Here's how the part is built. I have some questions about the finished solid (model axes, mm). A direction names the side the tool comes from. Round coordinates to 2 decimals unless told otherwise and drop trailing zeros. Loops run counter-clockwise (first coordinate to the right, second up) from the corner with the lowest first, then second, coordinate; pieces in that order, holes last. Notation, with made-up numbers: (42.5, -11.5) -> (90.5, -11.5) arc R15 cw to (90.5, 11.5) -> close; hole circle Ø8 at (13.25, -3.5). An arc over 180 degrees is marked (long way). One line per item, written item: value. Start each with the question number.
```python
from build123d import *

# Parameters (mm, degrees)
BOSS_EXTRUDE1_DEPTH = 8
SKETCH3_R           = 2.55
BOSS_EXTRUDE2_DEPTH = 1.5
CUT_EXTRUDE1_START  = -9.6
SKETCH3_3_R         = 2.55
CUT_EXTRUDE1_DEPTH  = 1.75


with BuildPart() as part:
    # Sketch1 → Boss-Extrude1 (new body)
    with BuildSketch(Plane(origin=(0, -47.198737708, 1.758e-06), x_dir=(1, 0, 0), z_dir=(1.517238059440084e-15, 0.9999999999999994, -3.725290356966477e-08))):
        with BuildLine():
            Line((7.999998093, 18.45445013), (7.999998093, 8.85445013))
            Line((7.999998093, 8.85445013), (14.894330873, 8.85445013))
            ThreePointArc((14.894330873, 8.85445013), (13.486635699, 16.156799215), (20.149998093, 12.85445013))
            ThreePointArc((20.149998093, 12.85445013), (19.302347178, 10.341087736), (17.105665312, 8.85445013))
            Line((17.105665312, 8.85445013), (23.999998093, 8.85445013))
            Line((23.999998093, 8.85445013), (23.999998093, 18.45445013))
            Line((23.999998093, 18.45445013), (7.999998093, 18.45445013))
        make_face()
    extrude(amount=BOSS_EXTRUDE1_DEPTH)

    # Sketch2 → Cut-Revolve1 (revolve, cut)
    with BuildSketch(Plane.ZY.offset(-15.999998093)):
        Polygon((-8.854448524, -44.263738058), (-8.619448462, -44.767697268), (-8.619448461, -44.798738029), (-8.854448524, -44.798738345), align=None)
    revolve(axis=Axis((15.999998093, -46.259040624, -12.929448669), (0, -1, 0)), mode=Mode.SUBTRACT)

    # Sketch3 → Boss-Extrude2 (add)
    with BuildSketch(Plane(origin=(0, -3.3e-07, -8.85445013), x_dir=(1, 0, 0), z_dir=(0, 3.725290356966478e-08, 0.9999999999999994))):
        with Locations(Location((11.999998093, -43.198737708, 0), (0, 0, 90))):
            Circle(SKETCH3_R)
        with Locations(Location((19.999998093, -43.198737708, 0), (0, 0, 90))):
            Circle(SKETCH3_R)
    extrude(amount=BOSS_EXTRUDE2_DEPTH)

    # Sketch3<3> → Cut-Extrude1 (cut)
    with BuildSketch(Plane(origin=(0, -3.3e-07, -8.85445013), x_dir=(1, 0, 0), z_dir=(0, 3.725290356966478e-08, 0.9999999999999994)).offset(CUT_EXTRUDE1_START)):
        with Locations(Location((11.999998093, -43.198737708, 0), (0, 0, 90))):
            Circle(SKETCH3_3_R)
        with Locations(Location((19.999998093, -43.198737708, 0), (0, 0, 90))):
            Circle(SKETCH3_3_R)
    extrude(amount=CUT_EXTRUDE1_DEPTH, mode=Mode.SUBTRACT)


solid = part.part
```
Q1. Will this pin go through, and if not, where does the flat tip stop? P1, Ø2.5, axis at x = 12, y = -43, coming from the -Z side.
Q2. Which directions (+Z, -Z, +X, -X, +Y, -Y) give clear straight access to the entire face, cutting with the end or side of a thin tool? Please do faces 1 (the flat face through (20, -43, -7.354)), 2 (the cylindrical face through (17.47, -43.53, -17.59)), 3 (the cylindrical face through (11.234, -40.766, -8.115)).
Q3. I want a section at D-D on x = 20.5. Please give me the cut outline in (y, z), plus the area to 3 significant figures.
Q4. If we mould it in two halves opening along Z, with no side actions, what happens to faces 4 (the flat face through (18, -47.199, -17)), 5 (the conical face through (15.83, -44.41, -17.07)), 6 (the flat face through (23, -43, -8.854))? For each: released by +Z, released by -Z, zero draft, split by the parting line, or undercut.
Q5. If I drill on line 1 along Z through (x, y) = (21.5, -42.75); line 2 along Z through (x, y) = (10.5, -40.25); line 3 along X through (y, z) = (-45.25, -11.25), over which ranges is the centre line in solid material (lowest first)?
Q6. I want a section at B-B on x = 9.75. Please give me the cut outline in (y, z).
Q7. I want a section at A-A on y = -43.5. Please give me the cut outline in (x, z).
Q8. I want a section at C-C on y = -41. Please give me the cut outline in (x, z).
Answers below:
1. P1: stops at z = -16.7
2. face 1: +Z, +X, -X, +Y, -Y
2. face 2: -Z
2. face 3: +Z
3. outline: (-47.2, -18.45) -> (-45.7, -18.45) -> (-45.7, -16.7) -> (-40.7, -16.7) -> (-40.7, -18.45) -> (-39.2, -18.45) -> (-39.2, -8.85) -> (-40.7, -8.85) -> (-40.7, -7.35) -> (-45.7, -7.35) -> (-45.7, -8.85) -> (-47.2, -8.85) -> close
3. area: 75.5 mm^2
4. face 4: zero draft
4. face 5: undercut
4. face 6: released by +Z
5. line 1: z = -16.7 to -7.35
5. line 2: z = -18.45 to -8.85
5. line 3: x = 8 to 12.17, 19.83 to 24
6. outline: (-47.2, -18.45) -> (-44.4, -18.45) -> (-44.4, -16.7) -> (-42, -16.7) -> (-42, -18.45) -> (-39.2, -18.45) -> (-39.2, -8.85) -> (-42, -8.85) -> (-42, -7.35) -> (-44.4, -7.35) -> (-44.4, -8.85) -> (-47.2, -8.85) -> close
7. outline: (8, -18.45) -> (9.47, -18.45) -> (9.47, -16.7) -> (14.45, -16.7) arc R4.15 cw to (14.89, -8.85) -> (14.53, -8.85) -> (14.53, -7.35) -> (9.47, -7.35) -> (9.47, -8.85) -> (8, -8.85) -> close; (14.53, -18.45) -> (17.47, -18.45) -> (17.47, -16.74) arc R4.15 cw to (14.53, -16.74) -> close; (17.11, -8.85) arc R4.15 cw to (17.55, -16.7) -> (22.53, -16.7) -> (22.53, -18.45) -> (24, -18.45) -> (24, -8.85) -> (22.53, -8.85) -> (22.53, -7.35) -> (17.47, -7.35) -> (17.47, -8.85) -> close
8. outline: (8, -18.45) -> (10.71, -18.45) -> (10.71, -16.7) -> (13.29, -16.7) -> (13.29, -18.45) -> (18.71, -18.45) -> (18.71, -16.7) -> (21.29, -16.7) -> (21.29, -18.45) -> (24, -18.45) -> (24, -8.85) -> (21.29, -8.85) -> (21.29, -7.35) -> (18.71, -7.35) -> (18.71, -8.85) -> (17.11, -8.85) arc R4.15 cw (long way) to (14.89, -8.85) -> (13.29, -8.85) -> (13.29, -7.35) -> (10.71, -7.35) -> (10.71, -8.85) -> (8, -8.85) -> close
